CAD build for the part. Positions are in the model's coordinates, mm. Coordinates: 2 decimals unless noted, no trailing zeros. Loops run counter-clockwise (first coordinate to the right, second up) from the corner with the lowest first, then second, coordinate; pieces in that order, holes last. Notation, with made-up numbers: (61.25, 83.25) -> (118.25, 83.25) arc R20 cw to (118.25, 98.25) -> close; hole circle Ø2 at (76.25, 37). An arc over 180 degrees is marked (long way). Write each question's results on one line, items separated by ' | '.
from build123d import *

# Parameters (mm, degrees)
SZKIC1_R                    = 0.6
DODANIE_WYCI_GNI_CIE1_DEPTH = 0.7


with BuildPart() as part:
    # Szkic1 → Dodanie-wyciągnięcie1 (new body)
    with BuildSketch(Plane.XY):
        with BuildLine():
            Line((0.8, -2.683281573), (0.8, -4.883281573))
            ThreePointArc((0.8, -4.883281573), (0.946446609, -5.236834964), (1.3, -5.383281573))
            Line((1.3, -5.383281573), (2.3, -5.383281573))
            ThreePointArc((2.3, -5.383281573), (2.653553391, -5.236834964), (2.8, -4.883281573))
            Line((2.8, -4.883281573), (2.8, -1.8))
            ThreePointArc((2.8, -1.8), (0, 3.8), (-2.8, -1.8))
            Line((-2.8, -1.8), (-2.8, -4.883281573))
            ThreePointArc((-2.8, -4.883281573), (-2.653553391, -5.236834964), (-2.3, -5.383281573))
            Line((-2.3, -5.383281573), (-1.3, -5.383281573))
            ThreePointArc((-1.3, -5.383281573), (-0.946446609, -5.236834964), (-0.8, -4.883281573))
            Line((-0.8, -4.883281573), (-0.8, -2.683281573))
            ThreePointArc((-0.8, -2.683281573), (0, 2.8), (0.8, -2.683281573))
        make_face()
        with Locations((1.8, -4.083281573)):
            Circle(SZKIC1_R, mode=Mode.SUBTRACT)
        with Locations(Location((-1.8, -4.083281573, 0), (0, 0, 180))):
            Circle(SZKIC1_R, mode=Mode.SUBTRACT)
    extrude(amount=DODANIE_WYCI_GNI_CIE1_DEPTH)


solid = part.part
1) Pin check, flat tips, straight feed: pin 1 (4 mm diameter, centred on x = 2, y = -0.5, fed in from -Z); pin 2 (0.7 mm diameter, centred on x = 1.8, y = -4.08, fed in from -Z). Stop position of each tip, or through.
Outcome:
pin 1: stops at z = 0 | pin 2: passes through
2) Slice it at D-D (x = 0). Write the cut outline in (y, z), then the cut area to 3 significant figures.
Outcome:
outline: (2.8, 0) -> (3.8, 0) -> (3.8, 0.7) -> (2.8, 0.7) -> close | area: 0.700 mm^2
3) Slice it at B-B (y = 0). Write the cut outline in (x, z), then the cut area to 3 significant figures.
Outcome:
outline: (-3.49, 0) -> (-2.8, 0) -> (-2.8, 0.7) -> (-3.49, 0.7) -> close; (2.8, 0) -> (3.49, 0) -> (3.49, 0.7) -> (2.8, 0.7) -> close | area: 0.962 mm^2
4) Slice it at A-A (x = 1.8). Write the cut outline in (y, z), then the cut area to 3 significant figures.
Outcome:
outline: (-5.38, 0) -> (-4.68, 0) -> (-4.68, 0.7) -> (-5.38, 0.7) -> close; (-3.48, 0) -> (-2.14, 0) -> (-2.14, 0.7) -> (-3.48, 0.7) -> close; (2.14, 0) -> (3.3, 0) -> (3.3, 0.7) -> (2.14, 0.7) -> close | area: 2.24 mm^2
5) Slice it at C-C (z = 0.6). Write the cut outline in (x, y).
Outcome:
outline: (-2.8, -4.88) arc R0.5 ccw to (-2.3, -5.38) -> (-1.3, -5.38) arc R0.5 ccw to (-0.8, -4.88) -> (-0.8, -2.68) arc R2.8 cw (long way) to (0.8, -2.68) -> (0.8, -4.88) arc R0.5 ccw to (1.3, -5.38) -> (2.3, -5.38) arc R0.5 ccw to (2.8, -4.88) -> (2.8, -1.8) arc R3.5 ccw (long way) to (-2.8, -1.8) -> close; hole circle Ø1.2 at (-1.8, -4.08); hole circle Ø1.2 at (1.8, -4.08)
6) Two-plate mould, pull along Y, no slides. Class faces 1 (the cylindrical face through (0.1, 3.8, 0.3)), 2 (the cylindrical face through (-0.1, 2.8, 0.3)), 3 (the flat face through (-1.6, -2.5, 0.7)): pulls with the +Y half, pulls with the -Y half, needs draft (parallel to the pull), parting line crosses it, or undercut.
Outcome:
face 1: parting line crosses it | face 2: undercut | face 3: needs draft
7) Drill centre lines: L1, parallel to Y at x = -2.25, z = 0.5; L2, parallel to X at y = -4.5, z = 0.35; L3, parallel to Y at x = -1.8, z = 0.2. Where is each one in solid material? Low to high. Write a range as from..to.
Outcome:
L1: y = -5.38..-4.48, -3.69..-1.67, 1.67..2.98 | L2: x = -2.8..-2.23, -1.37..-0.8, 0.8..1.37, 2.23..2.8 | L3: y = -5.38..-4.68, -3.48..-2.14, 2.14..3.3
